For this review, take the finished solid that the model builds, in its own axes (mm). A direction names the side the tool comes from. Coordinates: 2 decimals unless noted, no trailing zeros. Write each loop counter-clockwise with the first axis right and the second up, starting at its lowest first coordinate (ties: lowest second). Pieces come first, ordered by that corner, then holes. Notation, with made-up numbers: M -32,-8.5 L 9,-8.5 A20 cw 9,11.5 Z; hole C -13.75,18 d11. An arc over 180 degrees is marked long. One line per question, with ' | ' between items.
from build123d import *

# Parameters (mm, degrees)
CUT_EXTRUDE1_START = 9.78154
CUT_EXTRUDE1_DEPTH = 3.821845556


with BuildPart() as part:
    # Sketch2 → Revolve1 (revolve)
    with BuildSketch(Plane(origin=(0, 0, 0), x_dir=(0, 0, -1), z_dir=(1, 0, 0)), mode=Mode.PRIVATE) as revolve1_sk:
        with BuildLine():
            Line((-10.8077, 1.5875), (-10.8077, 2.2225))
            ThreePointArc((-10.8077, 2.2225), (-9.892752118, 3.57733025), (-8.605157143, 4.5847))
            Line((-8.605157143, 4.5847), (-8.2423, 4.5847))
            Line((-8.2423, 4.5847), (-8.2423, 2.413))
            Line((-8.2423, 2.413), (10.2123875, 2.413))
            Line((10.2123875, 2.413), (10.8077, 1.8176875))
            Line((10.8077, 1.8176875), (10.8077, 0))
            Line((10.8077, 0), (-8.864996448, 0))
            Line((-8.864996448, 0), (-9.78154, 1.5875))
            Line((-9.78154, 1.5875), (-10.8077, 1.5875))
        make_face()
    revolve(revolve1_sk.sketch.rotate(Axis((0, 0, 10.8077), (0, 0, -1)), 90), axis=Axis((0, 0, 10.8077), (0, 0, -1)))

    # Sketch3 → Cut-Extrude1 (cut, through all)
    with BuildSketch(Plane.XY.offset(CUT_EXTRUDE1_START)):
        Polygon((0, 1.833087105), (-1.5875, 0.916543552), (-1.5875, -0.916543552), (0, -1.833087105), (1.5875, -0.916543552), (1.5875, 0.916543552), align=None)
    extrude(amount=CUT_EXTRUDE1_DEPTH, mode=Mode.SUBTRACT)

    # Cut-Extrude2 cone 1 section (through the dimple's axis) → Cut-Extrude2 (revolve, cut)
    with BuildSketch(Plane(origin=(0, 0, 10.8077), x_dir=(0, -1, 0), z_dir=(1, 0, 0))):
        Polygon((0, 0), (1.833087105, 0), (0, 1.833087105), align=None)
    revolve(axis=Axis((0, 0, 10.8077), (0, 0, -1)), mode=Mode.SUBTRACT)


solid = part.part
1) We need section B-B on y = 3.75. State the section outline as (x, z) points.
Responses:
outline: M -2.64,8.24 L 2.64,8.24 L 2.64,8.61 A3.67 ccw -2.64,8.61 Z
2) Machinability: for faces 1 (the flat face through (0.783, -1.381, 10.173)), 2 (the flat face through (0, 0, -10.808)), 3 (the flat face through (2, 2, 8.242)), which of the approach directions +Z, -Z, +X, -X, +Y, -Y give a long, thin tool a straight path to every point of the face, cutting with its end or side? Answer none if there is none.
Responses:
face 1: +Z | face 2: -Z, +X, -X, +Y, -Y | face 3: -Z
3) We need section A-A on z = 1.25. State the section outline as (x, y) points, then the cut area to 3 significant figures.
Responses:
outline: C 0,0 d4.83 | area: 18.3 mm^2
4) To check wall thickness, follow line 1 along Z through (x, y) = (2.5, 1); line 2 along X through (y, z) = (1.25, -7); line 3 along X through (y, z) = (-1.75, -2.75). State the ranges of each line that lie inside material, in increasing order. Write a range as [from, to].
Responses:
line 1: [8.24, 10.56] | line 2: [-2.06, 2.06] | line 3: [-1.66, 1.66]
5) The part is to be moulded in two halves that separate along X. For faces 4 (the conical face through (0.26, -0.08, 9.02)), 5 (the flat face through (0, -2, 10.808)), 6 (the conical face through (-0.843, -1.486, 10.683)), 7 (the cylindrical face through (-0.994, 4.476, 8.421)), say which applies: +X half, -X half, draft (parallel to the pull), parting line (faces both ways), or undercut.
Responses:
face 4: undercut | face 5: draft | face 6: undercut | face 7: parting line
6) Insertion check: pin 1 Ø3 at (y, z) = (-1.5, -8) entering from +X; pin 2 Ø4 at (x, z) = (1.5, 6) entering from +Y; pin 3 Ø4 at (x, y) = (3, -1.5) entering from +Z; pin 4 Ø0.6 at (x, y) = (-1, -0.5) entering from +Z. Each pin has a flat end and moves straight along its axis. Give the tip position at first contact, or say it passes through.
Responses:
pin 1: x = 2.41 | pin 2: y = 2.41 | pin 3: z = 10.81 | pin 4: z = 9.68
